Design review of the part built by this model. Coordinates are the model's own, in mm. Give positions to 0.01 mm unless a question says otherwise; leave off trailing zeros. Order: outer loops, then holes, each group sorted by start corner. A loop starts at its lowest first (then second) coordinate and runs counter-clockwise, first axis right, second up. Notation, with made-up numbers: (14, 87.5) -> (52, 87.5) arc R30 cw to (52, 117.5) -> close; hole circle Ø8 at (14.25, 24). An arc over 180 degrees is marked (long way). One line per item, written item: value. Start each with the question number.
1) For pin 1 (8 mm diameter, centred on x = 3.5, y = 11, fed in from -Z); pin 2 (1 mm diameter, centred on x = 1, y = 57, fed in from -Z); pin 3 (0.9 mm diameter, centred on y = 22, z = 0.5, fed in from +X); pin 4 (0.5 mm diameter, centred on y = 9.5, z = 0.5, fed in from -X), all flat-tipped, find the tip position at first contact; note any pin that passes through.
2) Consider section A-A (y = 9.5). State the section outline as (x, z) points, plus the area to 3 significant figures.
3) Consider section B-B (x = -3). State how many separate pieces and enclosed holes the cut face has, plus the area to 3 significant figures.
4) Wall thickness on line 1 along Y through (x, z) = (-10.5, 1.1); line 2 along Y through (x, z) = (-11, 1.4); line 3 along X through (y, z) = (50, 0.35): over which ranges is each line inside the solid? List them lowest first. Write a range as from..to.
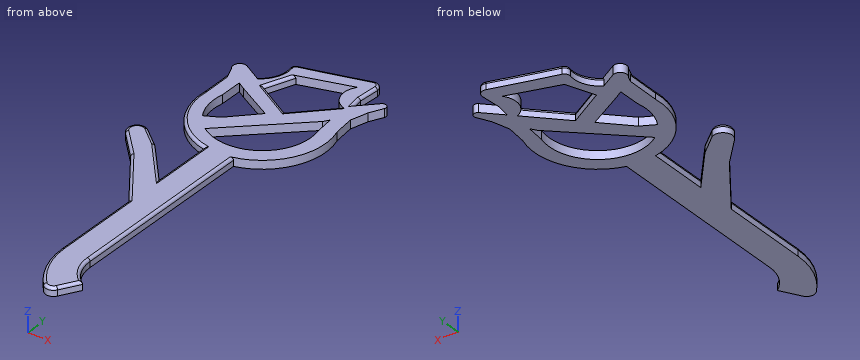
from build123d import *

# Parameters (mm, degrees)
F1_DEPTH = 1.5875
F2_R     = 0.508


with BuildPart() as f1:
    # F0 (on Top) → F1 (new body)
    with BuildSketch(Plane.XY):
        with BuildLine():
            Line((0, 0), (0, 36.181841))
            ThreePointArc((0, 36.181841), (7.365943, 42.068416), (8.157768, 51.46426))
            Line((8.157768, 51.46426), (7.721588, 55.367384))
            Line((7.721588, 55.367384), (8.652184, 58.648949))
            Line((8.652184, 58.648949), (9.870096, 61.084771))
            ThreePointArc((9.870096, 61.084771), (9.625521, 62.031582), (8.652184, 61.937326))
            Line((8.652184, 61.937326), (5.601979, 58.772682))
            Line((5.601979, 58.772682), (5.208922, 61.257325))
            Line((5.208922, 61.257325), (5.464944, 65.217614))
            ThreePointArc((5.464944, 65.217614), (4.987229, 66.294216), (3.830332, 66.515285))
            ThreePointArc((3.830332, 66.515285), (-2.071538, 64.775722), (-7.996314, 63.115845))
            ThreePointArc((-7.996314, 63.115845), (-8.59693, 62.663559), (-8.722139, 61.922193))
            ThreePointArc((-8.722139, 61.922193), (-9.034725, 58.886588), (-11.072643, 56.615136))
            Line((-11.072643, 56.615136), (-14.036038, 58.300966))
            ThreePointArc((-14.036038, 58.300966), (-15.610352, 57.989945), (-15.532072, 56.387113))
            Line((-15.532072, 56.387113), (-15.084018, 55.249624))
            Line((-15.084018, 55.249624), (-15.034714, 48.831713))
            ThreePointArc((-15.034714, 48.831713), (-12.693009, 40.514111), (-5.350228, 35.95893))
            Line((-5.350228, 35.95893), (-5.350228, 24.574336))
            Line((-5.350228, 24.574336), (-11.894111, 32.207083))
            Line((-11.894111, 32.207083), (-15.489053, 35.177361))
            ThreePointArc((-15.489053, 35.177361), (-17.791277, 34.799442), (-17.699574, 32.468208))
            Line((-17.699574, 32.468208), (-13.094822, 27.652631))
            Line((-13.094822, 27.652631), (-5.350228, 16.878592))
            Line((-5.350228, 16.878592), (-5.350228, 0))
            ThreePointArc((-5.350228, 0), (-4.344885, -5.247215), (-1.471247, -9.751234))
            ThreePointArc((-1.471247, -9.751234), (-0.189936, -10.218473), (0.952239, -9.473151))
            Line((0.952239, -9.473151), (3.04463, -5.891468))
            ThreePointArc((3.04463, -5.891468), (0.806147, -3.31584), (0, 0))
        make_face()
        with BuildLine():
            Line((-3.706487, 49.114973), (-8.372727, 44.273662))
            Line((-8.372727, 44.273662), (-10.95271, 42.896778))
            ThreePointArc((-10.95271, 42.896778), (-12.170993, 46.115262), (-12.113919, 49.556133))
            Line((-12.113919, 49.556133), (-12.113919, 53.752957))
            Line((-12.113919, 53.752957), (-10.684032, 52.888518))
            Line((-10.684032, 52.888518), (-3.706487, 49.114973))
        make_face(mode=Mode.SUBTRACT)
        with BuildLine():
            ThreePointArc((5.67868, 50.048354), (2.07604, 40.184885), (-8.42475, 40.206277))
            Line((-8.42475, 40.206277), (4.606551, 52.521817))
            Line((4.606551, 52.521817), (5.284048, 53.579681))
            Line((5.284048, 53.579681), (5.67868, 50.048354))
        make_face(mode=Mode.SUBTRACT)
        with BuildLine():
            Line((4.513334, 57.643192), (-1.646189, 51.252572))
            Line((-1.646189, 51.252572), (-8.593214, 55.204628))
            Line((-8.593214, 55.204628), (-6.536069, 60.575932))
            Line((-6.536069, 60.575932), (2.98464, 63.507594))
            ThreePointArc((2.98464, 63.507594), (2.320412, 60.203001), (4.513334, 57.643192))
        make_face(mode=Mode.SUBTRACT)
    extrude(amount=F1_DEPTH)

    # F2
    f2_edges = [f1.edges().sort_by_distance(p)[0] for p in [
        (-7.564642, 57.89028, 1.5875),
        (-5.119701, 53.2286, 1.5875),
        (1.433573, 54.447882, 1.5875),
        (-9.034725, 58.886588, 1.5875),
        (5.405451, 60.015003, 1.5875),
        (-15.059366, 52.040668, 1.5875),
        (-12.693009, 40.514111, 1.5875),
        (-5.350228, 30.266633, 1.5875),
        (-8.622169, 28.390709, 1.5875),
        (-13.691582, 33.692222, 1.5875),
        (-17.791277, 34.799442, 1.5875),
        (-15.397198, 30.060419, 1.5875),
        (-9.222525, 22.265611, 1.5875),
        (-5.350228, 8.439296, 1.5875),
        (0.806147, -3.31584, 1.5875),
    ]]
    fillet(f2_edges, radius=F2_R)


solid = f1.part
Checked values:
1. pin 1: stops at z = 0
1. pin 2: passes through
1. pin 3: stops at x = 0
1. pin 4: stops at x = -5.35
2. outline: (-5.35, 0) -> (0, 0) -> (0, 1.08) arc R0.51 ccw to (-0.51, 1.59) -> (-4.84, 1.59) arc R0.51 ccw to (-5.35, 1.08) -> close
2. area: 8.38 mm^2
3. separate pieces: 3
3. enclosed holes: 0
3. area: 88.5 mm^2
4. line 1: y = 24.04..30.58, 38.28..43.14, 52.79..57
4. line 2: y = 24.93..30.99, 38.85..42.97, 53.08..56.57
4. line 3: x = -15.04..-12.11, -5.34..1.94, 5.69..8.55
